from build123d import *

# Parameters (mm, degrees)
F1_DEPTH = 3
F2_W     = 1.4
F2_H     = 1.4
F3_DEPTH = 1.2
F4_R     = 0.5
F5_R     = 0.2
F6_W     = 0.8
F6_H     = 1
F7_DEPTH = 8


with BuildPart() as f1:
    # F0 (on Top) → F1 (new body)
    with BuildSketch(Plane.XY):
        Polygon((0, 0.8), (0, 0), (8, 0), (8, 0.8), (5.5, 0.8), (5.5, 3.3), (2.5, 3.3), (2.5, 0.8), align=None)
    extrude(amount=F1_DEPTH)

    # F2 (on face) → F3 (cut)
    with BuildSketch(Plane.XZ):
        with Locations((4, 1.5)):
            Rectangle(F2_W, F2_H)
    extrude(amount=-F3_DEPTH, mode=Mode.SUBTRACT)

    # F4
    f4_edges = [f1.edges().sort_by_distance(p)[0] for p in [
        (5.5, 2.05, 3),
        (2.5, 2.05, 3),
        (2.5, 2.05, 0),
        (5.5, 2.05, 0),
    ]]
    fillet(f4_edges, radius=F4_R)

    # F5
    f5_edges = [f1.edges().sort_by_distance(p)[0] for p in [
        (4, 3.3, 3),
        (5.353553, 3.3, 2.853553),
        (5.5, 3.3, 1.5),
        (5.353553, 3.3, 0.146447),
        (4, 3.3, 0),
        (2.646447, 3.3, 0.146447),
        (2.5, 3.3, 1.5),
        (2.646447, 3.3, 2.853553),
    ]]
    fillet(f5_edges, radius=F5_R)

    # F6 (on face) → F7 (join, through all)
    with BuildSketch(Plane.YZ.offset(8)):
        with Locations((0.4, 3.5)):
            Rectangle(F6_W, F6_H)
        with Locations((0.4, -0.5)):
            Rectangle(F6_W, F6_H)
    extrude(amount=-F7_DEPTH)


solid = f1.part
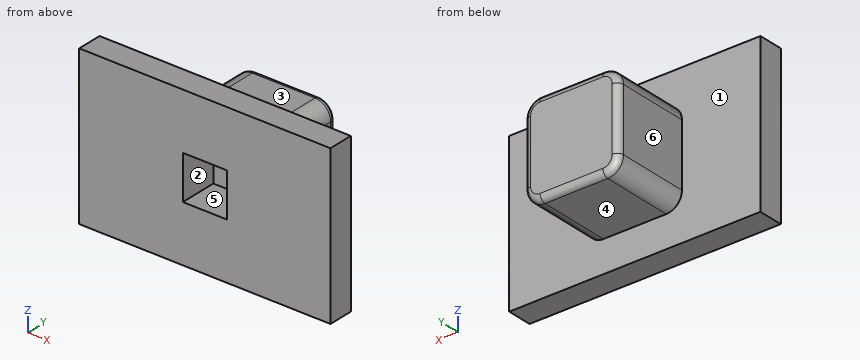
Work out the finished part from the listing and answer in its coordinate system (mm). Face numbers are marked on the shaded views. A direction names the side the tool comes from. Round coordinates to 2 decimals unless told otherwise and drop trailing zeros. Order: outer loops, then holes, each group sorted by start corner. A loop starts at its lowest first (then second) coordinate and runs counter-clockwise, first axis right, second up. Notation, with made-up numbers: M 53.5,27.25 L 83.5,27.25 A21 cw 83.5,47.25 Z; hole C -11,-8.75 d3. An arc over 180 degrees is marked long. Put each result on its own line as item: value. Start each with the question number.
Q1. Section A-A, the plane y = 0.9 is taken. Write down the section's boundary in (x, z).
Q2. Flat-ended cylindrical pins translate along their axes: pin 1 (1.6 mm diameter, centred on y = 2, z = 2, fed in from -X); pin 2 (0.7 mm diameter, centred on x = 4, z = 1.5, fed in from -Y); pin 3 (1.6 mm diameter, centred on y = 2, z = 1.5, fed in from +X). Find the tip coordinate at first contact, or state that the pin passes through.
Q3. Section C-C, the plane y = 2 is taken. Write down the section's boundary in (x, z), and give its area (3 significant figures).
Q4. Section D-D, the plane y = 0.45 is taken. Write down the section's boundary in (x, z), and give its area (3 significant figures).
Q5. Section B-B, the plane z = 0.9 is taken. Write down the section's boundary in (x, y), and give its area (3 significant figures).
Q6. Straight lines are drawn through the part: L1, parallel to Z at x = 4.5, y = 0.2; L2, parallel to X at y = 1.35, z = 2.25; L3, parallel to Z at x = 4, y = 2.05. For each, find the intervals that lie inside material, in ascending order. Write a range as [from, to].
Q7. For a pull along Z with two mould halves and no side action, classify the marked faces 1, 2 and 3 as pulls with the +Z half, pulls with the -Z half, needs draft (parallel to the pull), parting line crosses it, or undercut.
Q8. A tool of negligible diameter and unlimited length cuts with its end or side. For the marked faces 4, 5 and 6, from which of +Z, -Z, +X, -X, +Y, -Y can it reach the whole face along a straight path? Write none if from no direction.
Findings below:
1. outline: M 2.5,0.5 A0.5 ccw 3,0 L 5,0 A0.5 ccw 5.5,0.5 L 5.5,2.5 A0.5 ccw 5,3 L 3,3 A0.5 ccw 2.5,2.5 Z; hole M 3.3,0.8 L 4.7,0.8 L 4.7,2.2 L 3.3,2.2 Z
2. pin 1: stops at x = 2.5
2. pin 2: stops at y = 1.2
2. pin 3: stops at x = 5.5
3. outline: M 2.5,0.5 A0.5 ccw 3,0 L 5,0 A0.5 ccw 5.5,0.5 L 5.5,2.5 A0.5 ccw 5,3 L 3,3 A0.5 ccw 2.5,2.5 Z
3. area: 8.79 mm^2
4. outline: M 0,-1 L 8,-1 L 8,4 L 0,4 Z; hole M 3.3,0.8 L 4.7,0.8 L 4.7,2.2 L 3.3,2.2 Z
4. area: 38.0 mm^2
5. outline: M 0,0 L 3.3,0 L 3.3,1.2 L 4.7,1.2 L 4.7,0 L 8,0 L 8,0.8 L 5.5,0.8 L 5.5,3.1 A0.2 ccw 5.3,3.3 L 2.7,3.3 A0.2 ccw 2.5,3.1 L 2.5,0.8 L 0,0.8 Z
5. area: 12.2 mm^2
6. L1: z = [-1, 0.8], [2.2, 4]
6. L2: x = [2.5, 5.5]
6. L3: z = [0, 3]
7. face 1: needs draft
7. face 2: undercut
7. face 3: pulls with the +Z half
8. face 4: -Z, +X, -X, +Y
8. face 5: -Y
8. face 6: +Z, -Z, -X, +Y
